Read the model definition and answer for the solid it produces. Units are mm, in the model's axes. Face numbers are marked on the shaded views. Round coordinates to 2 decimals unless told otherwise and drop trailing zeros. Order: outer loops, then holes, each group sorted by start corner. A loop starts at its lowest first (then second) coordinate and runs counter-clockwise, first axis right, second up. Notation, with made-up numbers: (28, 82) - (79, 82) arc R17 ccw to (79, 107) - close; hole circle Ø5 at (-29, 2.25). An arc over 180 degrees is marked (long way). Put each result on its own line as item: value. Start each with the question number.
Q1. Each of these flat-tipped pins is pushed along its axis until it touches: pin 1 Ø3 at (y, z) = (5.5, 7) entering from -X; pin 2 Ø5 at (x, z) = (-15.5, 7.5) entering from +Y; pin 3 Ø1 at (y, z) = (-19, 2.5) entering from +X. Where does it stop, or does it pass through?
Q2. Section A-A on y = 0 is taken. Give the vertices of the cut face in (x, z), then the cut area to 3 significant figures.
Q3. For a pull along Y with two mould halves and no side action, classify the marked faces 1, 2 and 3 as pulls with the +Y half, pulls with the -Y half, needs draft (parallel to the pull), parting line crosses it, or undercut.
Q4. Find the intervals of material crossed by line 1 along Y through (x, z) = (0, 8.25); line 2 along Y through (x, z) = (0, 5); line 3 along X through (y, z) = (16, 9.5), in increasing order. Write a range as from..to.
Q5. Section C-C on z = 3.5 is taken. Give the vertices of the cut face in (x, y).
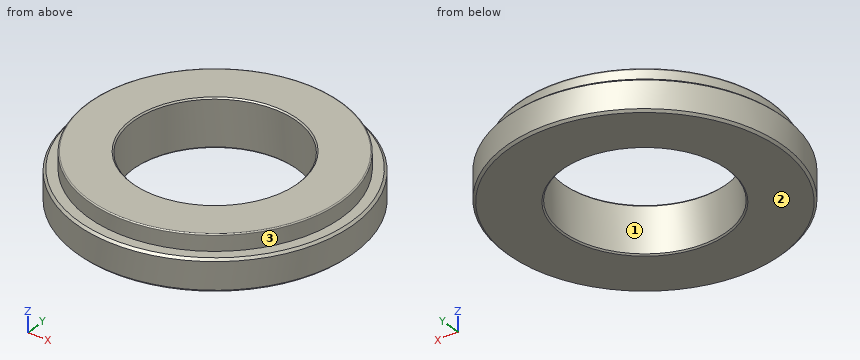
Autodesk Inventor part; units mm, degrees
ref_plane "YZ Plane" through (0, 0, 0) normal (1, 0, 0) x (0, 1, 0)
ref_plane "XZ Plane" through (0, 0, 0) normal (0, 1, 0) x (-1, 0, 0)
ref_plane "XY Plane" through (0, 0, 0) normal (0, 0, 1) x (1, 0, 0)
sketch "草圖1" plane through (0, 0, 0) normal (0, 0, 1) x (1, 0, 0)
  circle A0 centre (0, 0) radius 18.05
  circle A1 centre (0, 0) radius 30.65
  dimension "d0" = 36.1
  dimension "d1" = 61.3
extrude "擠出1" add sketch "草圖1" along normal blind 10.61
sketch "草圖2" plane through (0, 0, 10.61) normal (0, 0, 1) x (1, 0, 0)
  circle A0 centre (0, 0) radius 28
  circle A1 centre (0, 0) radius 39.6506
  dimension "d4" = 56
extrude "擠出2" cut sketch "草圖2" against normal blind 3.6
chamfer "倒角1" distance 0.3 angle 45 1 edges at (-18.05, 0, 0)
chamfer "倒角2" distance 0.5 angle 45 1 edges at (-30.65, 0, 0)
chamfer "倒角3" distance 0.5 angle 45 1 edges at (-30.65, 0, 7.01)
fillet "圓角1" radius 0.25 1 edges at (-28, 0, 10.61)
chamfer "倒角4" distance 0.3 angle 45 1 edges at (-18.05, 0, 10.61)
properties part number "IGX間隔環"
Findings:
1. pin 1: x = -30.38
1. pin 2: y = 27.66
1. pin 3: x = 24.44
2. outline: (-30.65, 0.5) - (-30.15, 0) - (-18.35, 0) - (-18.05, 0.3) - (-18.05, 10.31) - (-18.35, 10.61) - (-27.75, 10.61) arc R0.25 ccw to (-28, 10.36) - (-28, 7.01) - (-30.15, 7.01) - (-30.65, 6.51) - close; (18.05, 0.3) - (18.35, 0) - (30.15, 0) - (30.65, 0.5) - (30.65, 6.51) - (30.15, 7.01) - (28, 7.01) - (28, 10.36) arc R0.25 ccw to (27.75, 10.61) - (18.35, 10.61) - (18.05, 10.31) - close
2. area: 248 mm2
3. face 1: undercut
3. face 2: needs draft
3. face 3: parting line crosses it
4. line 1: -28..-18.05, 18.05..28
4. line 2: -30.65..-18.05, 18.05..30.65
4. line 3: -22.98..-8.35, 8.35..22.98
5. outline: circle Ø61.3 at (0, 0); hole circle Ø36.1 at (0, 0)
